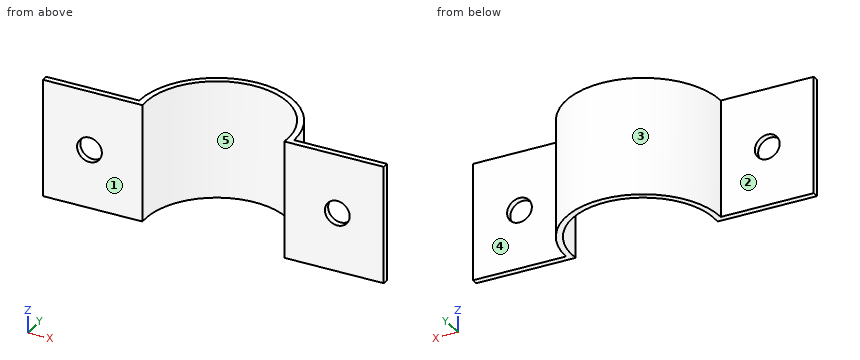
from build123d import *

# Parameters (mm, degrees)
Y_KSEKLIK_EKSTR_ZYON1_DEPTH = 19
IZIM2_R                     = 2
KES_EKSTR_ZYON1_DEPTH       = 19


with BuildPart() as part:
    # Çizim1 → Yükseklik-Ekstrüzyon1 (new body)
    with BuildSketch(Plane.XY):
        with BuildLine():
            Line((0, 0), (15, 0))
            ThreePointArc((15, 0), (27.5, 12.5), (40, 0))
            Line((40, 0), (55, 0))
            Line((55, 0), (55, -1))
            Line((55, -1), (38.956439237, -1))
            ThreePointArc((38.956439237, -1), (27.5, 11.5), (16.043560763, -1))
            Line((16.043560763, -1), (16, -1))
            Line((16, -1), (0, -1))
            Line((0, -1), (0, 0))
        make_face()
    extrude(amount=Y_KSEKLIK_EKSTR_ZYON1_DEPTH)

    # Çizim2 → Kes-Ekstrüzyon1 (cut)
    with BuildSketch(Plane(origin=(0, 0, 0), x_dir=(1, 0, 0), z_dir=(0, 1, 0))):
        with Locations(Location((7.5, -9.5, 0), (0, 0, 270))):
            Circle(IZIM2_R)
        with Locations(Location((47.5, -9.5, 0), (0, 0, 270))):
            Circle(IZIM2_R)
    extrude(amount=-KES_EKSTR_ZYON1_DEPTH, mode=Mode.SUBTRACT)


solid = part.part
Can you work these out from the model? Positions are in its coordinate system, mm. Face numbers are marked on the shaded views. A direction names the side the tool comes from. Give positions to 0.01 mm unless a question says otherwise; leave off trailing zeros. Order: outer loops, then holes, each group sorted by start corner. A loop starts at its lowest first (then second) coordinate and runs counter-clockwise, first axis right, second up. Notation, with made-up numbers: M 87.25,62.25 L 109.25,62.25 A26 ccw 109.25,98.25 Z; hole C 13,74.5 d6. An arc over 180 degrees is marked long. Use a Markdown table: item, result. Add a question column.
Item 1: Suppose I cut it at B-B (y = 7). List the corners of the cut face in (x, z) for me.
Item 2: Suppose I cut it at C-C (z = 8.75). List the corners of the cut face in (x, y) for me.
Item 3: We'd pull the mould along X, two halves only. Please class the marked faces 3, 4 and 5: +X half, -X half, draft (parallel to the pull), parting line (faces both ways), or undercut.
Item 4: If I drill on L1, parallel to X at y = -0.5, z = 9.5; L2, parallel to Y at x = 41, z = 9; L3, parallel to X at y = 6.75, z = 2.75, over which ranges is the centre line in solid material (lowest first)? Write a range as [from, to].
Item 5: Suppose I cut it at A-A (x = 7.5). List the corners of the cut face in (y, z) for me, then the cut area to 3 significant figures.
Item 6: For the marked faces 1 and 2, which set-ups out of +Z, -Z, +X, -X, +Y, -Y let a thin tool reach every point of the face, with its end or its side?
Item 7: Will these pins go through, and if not, where does the flat tip stop? pin 1 (1.5 mm diameter, centred on x = 23.5, z = 4.5, fed in from -Y); pin 2 (5 mm diameter, centred on x = 47.5, z = 9.5, fed in from +Y); pin 3 (1.5 mm diameter, centred on y = 3.5, z = 11.5, fed in from +X).
Item 8: Suppose I cut it at D-D (z = 4). List the corners of the cut face in (x, y) for me, then the cut area to 3 significant figures.
Answer sheet:
| question | item | result |
|---|---|---|
| 1 | outline | M 17.14,0 L 18.38,0 L 18.38,19 L 17.14,19 Z; M 36.62,0 L 37.86,0 L 37.86,19 L 36.62,19 Z |
| 2 | outline | M 0,-1 L 5.65,-1 L 5.65,0 L 0,0 Z; M 9.35,-1 L 16.04,-1 A11.5 cw long 38.96,-1 L 45.65,-1 L 45.65,0 L 40,0 A12.5 ccw 15,0 L 9.35,0 Z; M 49.35,-1 L 55,-1 L 55,0 L 49.35,0 Z |
| 3 | face 3 | parting line |
| 3 | face 4 | draft |
| 3 | face 5 | undercut |
| 4 | L1 | x = [0, 5.5], [9.5, 16.01], [38.99, 45.5], [49.5, 55] |
| 4 | L2 | y = [-1, 0] |
| 4 | L3 | x = [16.98, 18.19], [36.81, 38.02] |
| 5 | outline | M -1,0 L 0,0 L 0,7.5 L -1,7.5 Z; M -1,11.5 L 0,11.5 L 0,19 L -1,19 Z |
| 5 | area | 15.0 mm² |
| 6 | face 1 | +Z, -Z, +X, -X, -Y |
| 6 | face 2 | +Z, -Z, -X, +Y |
| 7 | pin 1 | stops at y = 10.47 |
| 7 | pin 2 | stops at y = 0 |
| 7 | pin 3 | stops at x = 39.69 |
| 8 | outline | M 0,-1 L 16.04,-1 A11.5 cw long 38.96,-1 L 55,-1 L 55,0 L 40,0 A12.5 ccw 15,0 L 0,0 Z |
| 8 | area | 69.7 mm² |
